For this review, use the dimensioned drawing (mm, ordinates from the lowest corner) and the shaded views. A direction names the side the tool comes from. Give positions to 0.01 mm unless a question says otherwise; leave off trailing zeros. Order: outer loops, then holes, each group sorted by start corner. A loop starts at its lowest first (then second) coordinate and runs counter-clockwise, first axis right, second up.
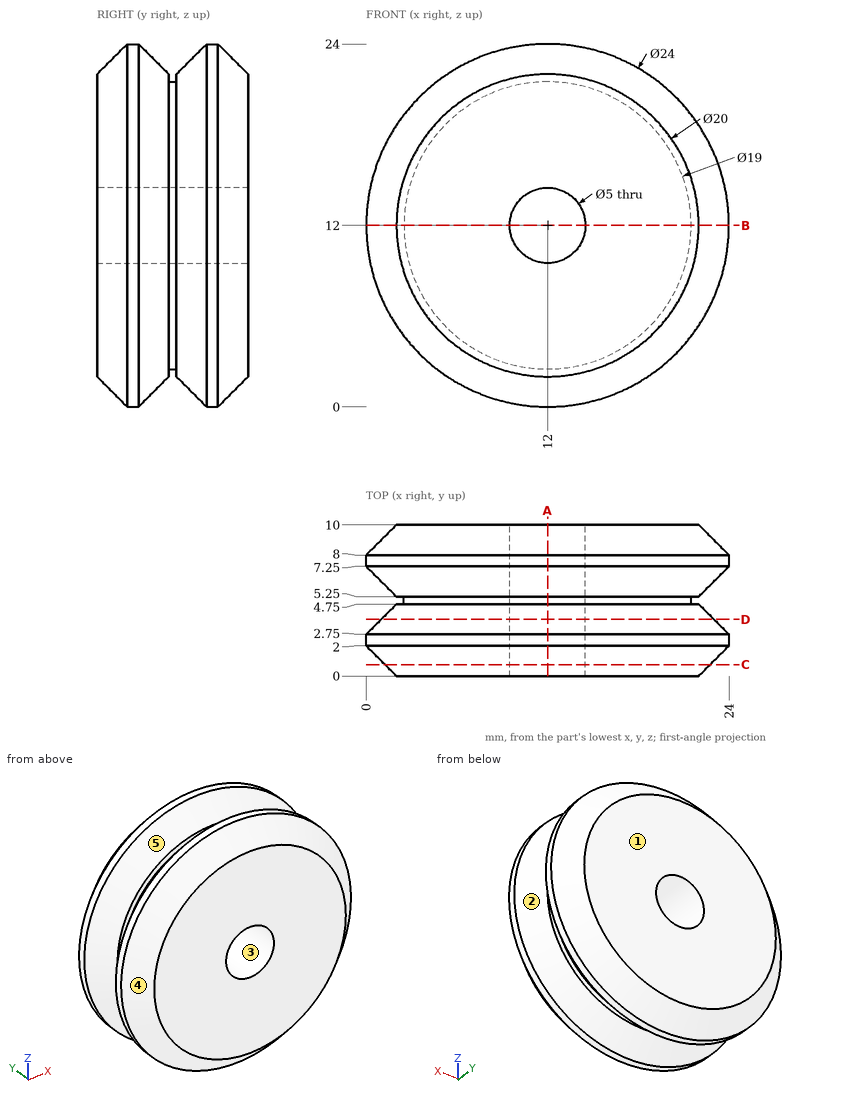
1. Take a section at B-B (z = 12). State the section outline as (x, y) points, then the cut area to 4 significant figures.
Recorded:
outline: (0, 2) - (2, 0) - (9.5, 0) - (9.5, 10) - (2, 10) - (0, 8) - (0, 7.25) - (2, 5.25) - (2.5, 5.25) - (2.5, 4.75) - (2, 4.75) - (0, 2.75) - close; (14.5, 0) - (22, 0) - (24, 2) - (24, 2.75) - (22, 4.75) - (21.5, 4.75) - (21.5, 5.25) - (22, 5.25) - (24, 7.25) - (24, 8) - (22, 10) - (14.5, 10) - close
area: 171.5 mm2
2. Machinability: for the marked faces 1 and 2, which of the approach directions +Z, -Z, +X, -X, +Y, -Y give a long, thin tool a straight path to every point of the face, cutting with its end or side? Answer none if there is none.
Recorded:
face 1: +Z, -Z, +X, -X, +Y
face 2: none
3. For line 1 along X through (y, z) = (5, 12); line 2 along X through (y, z) = (7.5, 12); line 3 along Z through (x, y) = (11.5, 0.75), list the stretches that pass through material, from the lowest coordinate up.
Recorded:
line 1: x = 2.5 to 9.5, 14.5 to 21.5
line 2: x = 0 to 9.5, 14.5 to 24
line 3: z = 1.26 to 9.55, 14.45 to 22.74
4. Take a section at D-D (y = 3.75). State the section outline as (x, z) points, then the cut area to 3 significant figures.
Recorded:
outline: circle Ø22 at (12, 12); hole circle Ø5 at (12, 12)
area: 360 mm2
5. Draft analysis for pull direction Y (two halves, no side actions). For the marked faces 3, 4 and 5, state which applies: pulls with the +Y half, pulls with the -Y half, needs draft (parallel to the pull), parting line crosses it, or undercut.
Recorded:
face 3: needs draft
face 4: pulls with the -Y half
face 5: undercut
6. Take a section at C-C (y = 0.75). State the section outline as (x, z) points.
Recorded:
outline: circle Ø21.5 at (12, 12); hole circle Ø5 at (12, 12)
7. For pin 1 (3 mm diameter, centred on x = 12, z = 12, fed in from +Y) (3 decimals); pin 2 (1 mm diameter, centred on y = 7.5, z = 17.5, fed in from +X); pin 3 (4 mm diameter, centred on x = 16, y = 4, fed in from +Z); pin 4 (1.5 mm diameter, centred on x = 19, y = 4.5, fed in from +Z), all flat-tipped, find the tip position at first contact; note any pin that passes through.
Recorded:
pin 1: passes through
pin 2: stops at x = 22.91
pin 3: stops at z = 23.75
pin 4: stops at z = 20.66
8. Take a section at A-A (x = 12). State the section outline as (y, z) points.
Recorded:
outline: (0, 2) - (2, 0) - (2.75, 0) - (4.75, 2) - (4.75, 2.5) - (5.25, 2.5) - (5.25, 2) - (7.25, 0) - (8, 0) - (10, 2) - (10, 9.5) - (0, 9.5) - close; (0, 14.5) - (10, 14.5) - (10, 22) - (8, 24) - (7.25, 24) - (5.25, 22) - (5.25, 21.5) - (4.75, 21.5) - (4.75, 22) - (2.75, 24) - (2, 24) - (0, 22) - close
